Verification items for the finished model (mm, model axes). A direction names the side the tool comes from. Round coordinates to 2 decimals unless told otherwise and drop trailing zeros. Write each loop counter-clockwise with the first axis right and the second up, starting at its lowest first coordinate (ties: lowest second). Pieces come first, ordered by that corner, then holes. Notation, with made-up numbers: (0.25, 5) - (52.25, 5) arc R24 ccw to (52.25, 23) - close; hole circle Ø1 at (-33, -34). An arc over 180 degrees is marked (long way). Write each question's results on one line, items separated by ' | '.
```python
from build123d import *

# Parameters (mm, degrees)
F0_W     = 92.541683
F0_H     = 58.561536
F1_DEPTH = 50.8
F2_W     = 84.106896
F2_H     = 48.43979
F3_DEPTH = 51.308
F4_W     = 25.545361
F4_H     = 22.773931
F5_DEPTH = 58.928
F6_R     = 6.504184
F7_DEPTH = 110.236


with BuildPart() as f1:
    # F0 (on Front) → F1 (new body)
    with BuildSketch(Plane.XZ):
        with Locations((1.566461, -7.229819)):
            Rectangle(F0_W, F0_H)
    extrude(amount=F1_DEPTH)

    # F2 (on Front) → F3 (cut)
    with BuildSketch(Plane.XZ):
        with Locations((1.445962, -7.711807)):
            Rectangle(F2_W, F2_H)
    extrude(amount=F3_DEPTH, mode=Mode.SUBTRACT)

    # F4 (on face) → F5 (cut)
    with BuildSketch(Plane.XY.offset(22.050949)):
        with Locations((3.253419, -11.386965)):
            Rectangle(F4_W, F4_H)
    extrude(amount=-F5_DEPTH, mode=Mode.SUBTRACT)

    # F6 (on face) → F7 (cut)
    with BuildSketch(Plane(origin=(-44.704381, 0, 0), x_dir=(0, -1, 0), z_dir=(-1, 0, 0))):
        with Locations((23.774298, -7.560832)):
            Circle(F6_R)
    extrude(amount=-F7_DEPTH, mode=Mode.SUBTRACT)


solid = f1.part
```
(1) Mould release check, pull along X, two halves, no side actions. Record for faces 4 (the flat face through (-2, -50.8, 17)), 5 (the flat face through (1, -25, 16.508)), 6 (the flat face through (47.837, -31, -8)): released by +X, released by -X, zero draft, split by the parting line, or undercut.
Answer:
face 4: zero draft | face 5: undercut | face 6: released by +X
(2) Section check D-D (y = -2.5). Record the cut outline in (x, z), plus the area to 3 significant figures.
Answer:
outline: (-44.7, -36.51) - (-9.52, -36.51) - (-9.52, -31.93) - (-40.61, -31.93) - (-40.61, 16.51) - (-9.52, 16.51) - (-9.52, 22.05) - (-44.7, 22.05) - close; (16.03, -36.51) - (47.84, -36.51) - (47.84, 22.05) - (16.03, 22.05) - (16.03, 16.51) - (43.5, 16.51) - (43.5, -31.93) - (16.03, -31.93) - close | area: 1,090 mm2
(3) Thickness scan on L1, parallel to Z at x = -35.5, y = -31; L2, parallel to X at y = -20, z = 17; L3, parallel to X at y = -45, z = 5.5. Record the ranges inside material, lowest first.
Answer:
L1: -36.51 to -31.93, 16.51 to 22.05 | L2: -44.7 to -9.52, 16.03 to 47.84 | L3: -44.7 to -40.61, 43.5 to 47.84
(4) Go/stop test with a flat-tipped pin: pin 1 Ø6 at (x, z) = (2, 18.5) entering from +Y. Record where the tip stops, or that it passes through.
Answer:
pin 1: y = -22.77
(5) Section check C-C (y = -39.5). Record the cut outline in (x, z).
Answer:
outline: (-44.7, -36.51) - (47.84, -36.51) - (47.84, 22.05) - (-44.7, 22.05) - close; hole (-40.61, -31.93) - (43.5, -31.93) - (43.5, 16.51) - (-40.61, 16.51) - close
(6) Section check B-B (z = 0.5). Record the cut outline in (x, y).
Answer:
outline: (-44.7, -50.8) - (-40.61, -50.8) - (-40.61, 0) - (-44.7, 0) - close; (43.5, -50.8) - (47.84, -50.8) - (47.84, 0) - (43.5, 0) - close
(7) Set-up check for faces 1 (the cylindrical face through (45.64, -22.36, -13.91)), 2 (the flat face through (43.499, -31, -8)), 3 (the flat face through (3, -22.774, 19)): record each of +Z, -Z, +X, -X, +Y, -Y from which the full face is reachable in a straight line by a thin tool's end or side.
Answer:
face 1: +X, -X | face 2: +Y, -Y | face 3: +Z, -Z, +Y
(8) Section check A-A (x = 5.5). Record the cut outline in (y, z).
Answer:
outline: (-50.8, -36.51) - (-22.77, -36.51) - (-22.77, -31.93) - (-50.8, -31.93) - close; (-50.8, 16.51) - (-22.77, 16.51) - (-22.77, 22.05) - (-50.8, 22.05) - close
